Model file for the job. Use its own axes, mm. A direction names the side the tool comes from. Round coordinates to 2 decimals unless told otherwise and drop trailing zeros. Order: outer loops, then holes, each group sorted by start corner. A loop starts at its lowest first (then second) coordinate and runs counter-clockwise, first axis right, second up. Notation, with made-up numbers: (49.25, 48) - (61.25, 48) arc R33 cw to (61.25, 76) - close; hole circle Ø9 at (47.25, -35). An arc over 180 degrees is marked (long way). Use one line per item in the form item = value.
from build123d import *

# Parameters (mm, degrees)
BASE_FLANGE1_DEPTH = 76
SKETCH2_R          = 3
CUT_EXTRUDE1_DEPTH = 843.237234988
SKETCH3_R          = 3
CUT_EXTRUDE2_DEPTH = 10


# Read off the part's stored shape, not the designer's step: Base-Flange1
with BuildPart() as part:
    # Base-Flange1 outline → Base-Flange1 (new body)
    with BuildSketch(Plane(origin=(0, 0, 0), x_dir=(1, 0, 0), z_dir=(0, 1, 0))):
        with BuildLine():
            Line((822.7, 144), (822.7, 0))
            Line((822.7, 0), (823.4, 0))
            Line((823.4, 0), (823.4, 144))
            ThreePointArc((823.4, 144), (818.713708499, 155.313708499), (807.4, 160))
            Line((807.4, 160), (16, 160))
            ThreePointArc((16, 160), (4.686291501, 155.313708499), (0, 144))
            Line((0, 144), (0, 0))
            Line((0, 0), (0.7, 0))
            Line((0.7, 0), (0.7, 144))
            ThreePointArc((0.7, 144), (5.181266248, 154.818733752), (16, 159.3))
            Line((16, 159.3), (807.4, 159.3))
            ThreePointArc((807.4, 159.3), (818.218733752, 154.818733752), (822.7, 144))
        make_face()
    extrude(amount=BASE_FLANGE1_DEPTH)

    # Sketch2 → Cut-Extrude1 (cut, through all)
    with BuildSketch(Plane(origin=(823.4, 0, 0), x_dir=(0, 0, -1), z_dir=(1, 0, 0))):
        with Locations((16, 70)):
            Circle(SKETCH2_R)
        with Locations((111, 70)):
            Circle(SKETCH2_R)
        with Locations(Location((111, 6, 0), (0, 0, 180))):
            Circle(SKETCH2_R)
        with Locations(Location((16, 6, 0), (0, 0, 180))):
            Circle(SKETCH2_R)
    extrude(amount=-CUT_EXTRUDE1_DEPTH, mode=Mode.SUBTRACT)

    # Sketch3 → Cut-Extrude2 (cut)
    with BuildSketch(Plane(origin=(0, 0, -160), x_dir=(-1, 0, 0), z_dir=(0, 0, -1))):
        with Locations((-762.4, 70)):
            Circle(SKETCH3_R)
        with Locations((-582.4, 70)):
            Circle(SKETCH3_R)
        with Locations((-402.4, 70)):
            Circle(SKETCH3_R)
        with Locations((-222.4, 70)):
            Circle(SKETCH3_R)
        with Locations((-42.4, 70)):
            Circle(SKETCH3_R)
        with Locations((137.6, 70)):
            Circle(SKETCH3_R)
        with Locations((317.6, 70)):
            Circle(SKETCH3_R)
        with Locations((317.6, 6)):
            Circle(SKETCH3_R)
        with Locations((137.6, 6)):
            Circle(SKETCH3_R)
        with Locations((-42.4, 6)):
            Circle(SKETCH3_R)
        with Locations((-222.4, 6)):
            Circle(SKETCH3_R)
        with Locations((-402.4, 6)):
            Circle(SKETCH3_R)
        with Locations((-582.4, 6)):
            Circle(SKETCH3_R)
        with Locations((-762.4, 6)):
            Circle(SKETCH3_R)
    extrude(amount=-CUT_EXTRUDE2_DEPTH, mode=Mode.SUBTRACT)


solid = part.part
(1) Slice it at A-A on z = -38.5. Give the cut face in (x, y), then the cut area to 3 significant figures.
Report:
outline = (0, 0) - (0.7, 0) - (0.7, 76) - (0, 76) - close; (822.7, 0) - (823.4, 0) - (823.4, 76) - (822.7, 76) - close
area = 106 mm2
(2) Slice it at B-B on y = 54.5. Give the cut face in (x, z).
Report:
outline = (0, -144) arc R16 ccw to (16, -160) - (807.4, -160) arc R16 ccw to (823.4, -144) - (823.4, 0) - (822.7, 0) - (822.7, -144) arc R15.3 cw to (807.4, -159.3) - (16, -159.3) arc R15.3 cw to (0.7, -144) - (0.7, 0) - (0, 0) - close
(3) Probe probe 1 along Y at (x, z) = (0.5, -16); probe 2 along X at (y, z) = (48.5, -97); probe 3 along Z at (x, y) = (287, 4). List the from-to ranges inside material, lowest first. Write a range as [from, to].
Report:
probe_1 = [0, 3], [9, 67], [73, 76]
probe_2 = [0, 0.7], [822.7, 823.4]
probe_3 = [-160, -159.3]
(4) Tool access for faces 1 (the face through (5.063, 37.468, -154.699)), 2 (the face through (818.837, 37.468, -155.189)): list every direction of +Z, -Z, +X, -X, +Y, -Y with a clear straight run to the whole face (end or side of a thin tool).
Report:
face_1 = +Z, +Y, -Y
face_2 = -Z, +X, +Y, -Y
(5) Slice it at C-C on x = 65. Give the cut face in (y, z), then the cut area to 3 significant figures.
Report:
outline = (0, -160) - (76, -160) - (76, -159.3) - (0, -159.3) - close
area = 53.2 mm2
(6) Pin check, flat tips, straight feed: pin 1 (5 mm diameter, centred on x = 762.4, y = 6, fed in from -Z); pin 2 (8 mm diameter, centred on x = 212.5, y = 39.5, fed in from +Z). Stop position of each tip, or through.
Report:
pin_1 = through
pin_2 = -159.3
